```python
from build123d import *

# Parameters (mm, degrees)
SKETCH_1_W          = 206
SKETCH_1_H          = 84
EXTRUDE_1_DEPTH     = 5.8
CUT_EXTRUDE_1_REACH = 224.544
SKETCH_2_R          = 4


with BuildPart() as part:
    # Эскиз1 → Бобышка-Вытянуть1 (new body)
    with BuildSketch(Plane.XY):
        with Locations((103, 42)):
            Rectangle(SKETCH_1_W, SKETCH_1_H)
        with BuildLine():
            Line((22, 62), (22, 22))
            ThreePointArc((22, 22), (18, 18), (14, 22))
            Line((14, 22), (14, 62))
            ThreePointArc((14, 62), (18, 66), (22, 62))
        make_face(mode=Mode.SUBTRACT)
        with BuildLine():
            Line((107, 62), (107, 22))
            ThreePointArc((107, 22), (103, 18), (99, 22))
            Line((99, 22), (99, 62))
            ThreePointArc((99, 62), (103, 66), (107, 62))
        make_face(mode=Mode.SUBTRACT)
        with BuildLine():
            Line((192, 62), (192, 22))
            ThreePointArc((192, 22), (188, 18), (184, 22))
            Line((184, 22), (184, 62))
            ThreePointArc((184, 62), (188, 66), (192, 62))
        make_face(mode=Mode.SUBTRACT)
    extrude(amount=EXTRUDE_1_DEPTH)

    # Эскиз2 → Вырез-Вытянуть1 (cut, up to next)
    with BuildSketch(Plane.XY.offset(5.8), mode=Mode.PRIVATE) as cut_extrude_1_sk1:
        with Locations((60.5, 67)):
            Circle(SKETCH_2_R)
    cut_extrude_1_tool1 = extrude(cut_extrude_1_sk1.sketch, amount=-CUT_EXTRUDE_1_REACH, mode=Mode.PRIVATE) & part.part
    # Эскиз2 → Вырез-Вытянуть1 (cut, up to next)
    with BuildSketch(Plane.XY.offset(5.8), mode=Mode.PRIVATE) as cut_extrude_1_sk2:
        with Locations((60.5, 17)):
            Circle(SKETCH_2_R)
    cut_extrude_1_tool2 = extrude(cut_extrude_1_sk2.sketch, amount=-CUT_EXTRUDE_1_REACH, mode=Mode.PRIVATE) & part.part
    # Эскиз2 → Вырез-Вытянуть1 (cut, up to next)
    with BuildSketch(Plane.XY.offset(5.8), mode=Mode.PRIVATE) as cut_extrude_1_sk3:
        with Locations((145.5, 17)):
            Circle(SKETCH_2_R)
    cut_extrude_1_tool3 = extrude(cut_extrude_1_sk3.sketch, amount=-CUT_EXTRUDE_1_REACH, mode=Mode.PRIVATE) & part.part
    # Эскиз2 → Вырез-Вытянуть1 (cut, up to next)
    with BuildSketch(Plane.XY.offset(5.8), mode=Mode.PRIVATE) as cut_extrude_1_sk4:
        with Locations((145.5, 67)):
            Circle(SKETCH_2_R)
    cut_extrude_1_tool4 = extrude(cut_extrude_1_sk4.sketch, amount=-CUT_EXTRUDE_1_REACH, mode=Mode.PRIVATE) & part.part
    add(cut_extrude_1_tool1.solids().sort_by_distance((60.5, 67, 5.8))[0], mode=Mode.SUBTRACT)
    add(cut_extrude_1_tool2.solids().sort_by_distance((60.5, 17, 5.8))[0], mode=Mode.SUBTRACT)
    add(cut_extrude_1_tool3.solids().sort_by_distance((145.5, 17, 5.8))[0], mode=Mode.SUBTRACT)
    add(cut_extrude_1_tool4.solids().sort_by_distance((145.5, 67, 5.8))[0], mode=Mode.SUBTRACT)


solid = part.part
```
Geometry: final body of the model. Coordinates: model frame, mm. A direction names the side the tool comes from. Round coordinates to 2 decimals unless told otherwise and drop trailing zeros. Order: outer loops, then holes, each group sorted by start corner. A loop starts at its lowest first (then second) coordinate and runs counter-clockwise, first axis right, second up. Notation, with made-up numbers: (27, 74.25) - (40, 74.25) arc R27 cw to (40, 102.25) - close; hole circle Ø2 at (16, -32). An arc over 180 degrees is marked (long way). Use CSV: the item, a comma, the result in double quotes. Start each with the question number.
Q1. Mould query, pull axis X, two halves, no side actions, for faces 3 (the face through (102, 0, 3)), 4 (the face through (0, 41, 3)), 5 (the face through (103, 18, 3)). Classes: +X half, -X half, draft (parallel to the pull), parting line (faces both ways), or undercut.
Q2. Section query B-B (y = 54). Return loops of the section in (x, z), and give its area (3 significant figures).
Q3. Access query for faces 1 (the face through (79, 43, 5.8)), 2 (the face through (188, 66, 3)). Directions: +Z, -Z, +X, -X, +Y, -Y. A direction counts if a zero-diameter tool reaches every point of the face in a straight line with its end or side. Return the directions, or none.
Q4. Section query D-D (z = 2.8). Return loops of the section in (x, y).
Q5. Section query A-A (x = 145.5). Return loops of the section in (y, z), and give its area (3 significant figures).
Q6. First-contact query: pin 1 (5 mm diameter, centred on x = 145.5, y = 67, fed in from -Z). Flat tip, straight axial feed; report the tip coordinate or a pass-through.
Q7. Section query C-C (x = 103). Return loops of the section in (y, z), and give its area (3 significant figures).
Q8. Material intervals for line 1 along Y through (x, z) = (60.5, 0.7); line 2 along X through (y, z) = (62, 4.9), sorted ascending. Write a range as from..to.
Result set:
1,face 3,"draft"
1,face 4,"-X half"
1,face 5,"undercut"
2,outline,"(0, 0) - (14, 0) - (14, 5.8) - (0, 5.8) - close; (22, 0) - (99, 0) - (99, 5.8) - (22, 5.8) - close; (107, 0) - (184, 0) - (184, 5.8) - (107, 5.8) - close; (192, 0) - (206, 0) - (206, 5.8) - (192, 5.8) - close"
2,area,"1,060 mm2"
3,face 1,"+Z, +X, -X, +Y, -Y"
3,face 2,"+Z, -Z"
4,outline,"(0, 0) - (206, 0) - (206, 84) - (0, 84) - close; hole (14, 22) arc R4 ccw to (22, 22) - (22, 62) arc R4 ccw to (14, 62) - close; hole circle Ø8 at (60.5, 17); hole circle Ø8 at (60.5, 67); hole (99, 22) arc R4 ccw to (107, 22) - (107, 62) arc R4 ccw to (99, 62) - close; hole circle Ø8 at (145.5, 17); hole circle Ø8 at (145.5, 67); hole (184, 22) arc R4 ccw to (192, 22) - (192, 62) arc R4 ccw to (184, 62) - close"
5,outline,"(0, 0) - (13, 0) - (13, 5.8) - (0, 5.8) - close; (21, 0) - (63, 0) - (63, 5.8) - (21, 5.8) - close; (71, 0) - (84, 0) - (84, 5.8) - (71, 5.8) - close"
5,area,"394 mm2"
6,pin 1,"passes through"
7,outline,"(0, 0) - (18, 0) - (18, 5.8) - (0, 5.8) - close; (66, 0) - (84, 0) - (84, 5.8) - (66, 5.8) - close"
7,area,"209 mm2"
8,line 1,"y = 0..13, 21..63, 71..84"
8,line 2,"x = 0..14, 22..99, 107..184, 192..206"
